Here's how the part is built. I have some questions about the finished solid (model axes, mm). A direction names the side the tool comes from. Round coordinates to 2 decimals unless told otherwise and drop trailing zeros. Write each loop counter-clockwise with the first axis right and the second up, starting at its lowest first coordinate (ties: lowest second). Pieces come first, ordered by that corner, then holes. Notation, with made-up numbers: (77.25, 71) - (132.25, 71) arc R23 cw to (132.25, 84) - close; hole circle Ø10 at (-38, 66.25). An arc over 180 degrees is marked (long way). One line per item, written item: value. Start each with the question number.
Item 1: For P1, Ø4.5, axis at y = 2, z = 23, coming from the -X side; P2, Ø2, axis at y = 0.5, z = 43, coming from the +X side; P3, Ø3, axis at y = 2, z = 32.5, coming from the +X side, each with a flat end and sliding along its axis, tell me the tip position at first contact or that it passes through.
Item 2: Imagine slicing it at B-B, the plane x = 27. Please give me the cut outline in (y, z).
Item 3: Imagine slicing it at C-C, the plane z = 41.5. Please give me the cut outline in (x, y), then the cut area to 3 significant figures.
Item 4: Imagine slicing it at D-D, the plane z = 8.5. Please give me the cut outline in (x, y).
Item 5: Thinking about a two-plate mould opening in X: for faces 4 (the face through (-18, 2, 45)), 5 (the face through (-20, 2, 27)), 6 (the face through (-79, 0, 27)), 7 (the face through (79, 0, 27)), which applies, released by +X, released by -X, zero draft, split by the parting line, or undercut?
Item 6: For faces 1 (the face through (1, 2, 5)), 2 (the face through (-15, 2, 27)), 3 (the face through (-1, 0, 55)), which set-ups out of +Z, -Z, +X, -X, +Y, -Y let a thin tool reach every point of the face, with its end or its side?
Item 7: Imagine slicing it at A-A, the plane y = 2.25. Please give me the cut outline in (x, z), then the cut area to 3 significant figures.
Item 8: If I drill on line 1 (Z direction, x = -52.5, y = 3.25); line 2 (X direction, y = 1.5, z = 12); line 3 (X direction, y = 2, z = 32), over which ranges is the centre line in solid material (lowest first)?
```python
from build123d import *

# Parameters (mm, degrees)
F1_DEPTH = 55
F2_W     = 4
F2_H     = 5
F3_DEPTH = 83
F4_W     = 5
F4_H     = 35
F5_DEPTH = 4


with BuildPart() as f1:
    # F0 (on Top) → F1 (new body)
    with BuildSketch(Plane.XY):
        Polygon((-75, 4), (-83, -4), (83, -4), (75, 4), align=None)
    extrude(amount=F1_DEPTH)

    # F2 (on Right) → F3 (cut, symmetric)
    with BuildSketch(Plane.YZ):
        with Locations((2, 7.5)):
            Rectangle(F2_W, F2_H)
    extrude(amount=F3_DEPTH, both=True, mode=Mode.SUBTRACT)

    # F4 (on Front) → F5 (cut)
    with BuildSketch(Plane.XZ):
        with Locations((-17.5, 27.5)):
            Rectangle(F4_W, F4_H)
    extrude(amount=-F5_DEPTH, mode=Mode.SUBTRACT)


solid = f1.part
```
Values follow:
1. P1: stops at x = -79.25
1. P2: stops at x = 79.5
1. P3: stops at x = 78.5
2. outline: (-4, 0) - (4, 0) - (4, 5) - (0, 5) - (0, 10) - (4, 10) - (4, 55) - (-4, 55) - close
3. outline: (-83, -4) - (83, -4) - (75, 4) - (-15, 4) - (-15, 0) - (-20, 0) - (-20, 4) - (-75, 4) - close
3. area: 1,240 mm^2
4. outline: (-83, -4) - (83, -4) - (79, 0) - (-79, 0) - close
5. face 4: undercut
5. face 5: undercut
5. face 6: released by -X
5. face 7: released by +X
6. face 1: +X, -X, +Y
6. face 2: +Y
6. face 3: +Z, +X, -X, +Y, -Y
7. outline: (-76.75, 0) - (76.75, 0) - (76.75, 5) - (-76.75, 5) - close; (-76.75, 10) - (-20, 10) - (-20, 45) - (-15, 45) - (-15, 10) - (76.75, 10) - (76.75, 55) - (-76.75, 55) - close
7. area: 7,500 mm^2
8. line 1: z = 0 to 5, 10 to 55
8. line 2: x = -77.5 to -20, -15 to 77.5
8. line 3: x = -77 to -20, -15 to 77
